Geometry check sheet. Reference: the model listing, model coordinates, mm. Coordinates: 2 decimals unless noted, no trailing zeros. Write each loop counter-clockwise with the first axis right and the second up, starting at its lowest first coordinate (ties: lowest second). Pieces come first, ordered by that corner, then holes. Notation, with made-up numbers: (16, -29.75) -> (27, -29.75) arc R19 ccw to (27, 3.25) -> close; hole circle Ø8 at (53, 66.25). An arc over 180 degrees is marked (long way). One line per question, with ' | ' between items.
from build123d import *

# Parameters (mm, degrees)
F0_W     = 152.4
F0_H     = 114.3
F0_R     = 9.525
F1_DEPTH = 6.35
F2_R     = 12.7


with BuildPart() as f1:
    # F0 (on Top) → F1 (new body)
    with BuildSketch(Plane.XY):
        Rectangle(F0_W, F0_H)
        with BuildLine():
            Line((-8.885304, -47.623662), (-9.393304, -47.623662))
            Line((-9.393304, -47.623662), (-59.177304, -47.623662))
            ThreePointArc((-59.177304, -47.623662), (-59.307662, -47.626338), (-59.43802, -47.623662))
            Line((-59.43802, -47.623662), (-59.685304, -47.623662))
            ThreePointArc((-59.685304, -47.623662), (-59.815662, -47.626338), (-59.94602, -47.623662))
            Line((-59.94602, -47.623662), (-60.193304, -47.623662))
            ThreePointArc((-60.193304, -47.623662), (-63.499331, -44.515193), (-60.323662, -41.273662))
            Line((-60.323662, -41.273662), (-59.815662, -41.273662))
            Line((-59.815662, -41.273662), (-59.307662, -41.273662))
            Line((-59.307662, -41.273662), (-9.393304, -41.273662))
            Line((-9.393304, -41.273662), (-8.885304, -41.273662))
            Line((-8.885304, -41.273662), (-8.377304, -41.273662))
            ThreePointArc((-8.377304, -41.273662), (-5.202304, -44.448662), (-8.377304, -47.623662))
            Line((-8.377304, -47.623662), (-8.885304, -47.623662))
        make_face(mode=Mode.SUBTRACT)
        with BuildLine():
            Line((-8.885304, -34.923662), (-9.393304, -34.923662))
            Line((-9.393304, -34.923662), (-59.177304, -34.923662))
            ThreePointArc((-59.177304, -34.923662), (-59.307662, -34.926338), (-59.43802, -34.923662))
            Line((-59.43802, -34.923662), (-59.685304, -34.923662))
            ThreePointArc((-59.685304, -34.923662), (-59.815662, -34.926338), (-59.94602, -34.923662))
            Line((-59.94602, -34.923662), (-60.193304, -34.923662))
            ThreePointArc((-60.193304, -34.923662), (-63.499331, -31.815193), (-60.323662, -28.573662))
            Line((-60.323662, -28.573662), (-59.815662, -28.573662))
            Line((-59.815662, -28.573662), (-59.307662, -28.573662))
            Line((-59.307662, -28.573662), (-9.393304, -28.573662))
            Line((-9.393304, -28.573662), (-8.885304, -28.573662))
            Line((-8.885304, -28.573662), (-8.377304, -28.573662))
            ThreePointArc((-8.377304, -28.573662), (-5.202304, -31.748662), (-8.377304, -34.923662))
            Line((-8.377304, -34.923662), (-8.885304, -34.923662))
        make_face(mode=Mode.SUBTRACT)
        with BuildLine():
            Line((-8.885304, -22.223662), (-9.393304, -22.223662))
            Line((-9.393304, -22.223662), (-59.177304, -22.223662))
            ThreePointArc((-59.177304, -22.223662), (-59.307662, -22.226338), (-59.43802, -22.223662))
            Line((-59.43802, -22.223662), (-59.685304, -22.223662))
            ThreePointArc((-59.685304, -22.223662), (-59.815662, -22.226338), (-59.94602, -22.223662))
            Line((-59.94602, -22.223662), (-60.193304, -22.223662))
            ThreePointArc((-60.193304, -22.223662), (-63.499331, -19.115193), (-60.323662, -15.873662))
            Line((-60.323662, -15.873662), (-59.815662, -15.873662))
            Line((-59.815662, -15.873662), (-59.307662, -15.873662))
            Line((-59.307662, -15.873662), (-9.393304, -15.873662))
            Line((-9.393304, -15.873662), (-8.885304, -15.873662))
            Line((-8.885304, -15.873662), (-8.377304, -15.873662))
            ThreePointArc((-8.377304, -15.873662), (-5.202304, -19.048662), (-8.377304, -22.223662))
            Line((-8.377304, -22.223662), (-8.885304, -22.223662))
        make_face(mode=Mode.SUBTRACT)
        with BuildLine():
            Line((-8.885304, -9.523662), (-9.393304, -9.523662))
            Line((-9.393304, -9.523662), (-59.177304, -9.523662))
            ThreePointArc((-59.177304, -9.523662), (-59.307662, -9.526338), (-59.43802, -9.523662))
            Line((-59.43802, -9.523662), (-59.685304, -9.523662))
            ThreePointArc((-59.685304, -9.523662), (-59.815662, -9.526338), (-59.94602, -9.523662))
            Line((-59.94602, -9.523662), (-60.193304, -9.523662))
            ThreePointArc((-60.193304, -9.523662), (-63.499331, -6.415193), (-60.323662, -3.173662))
            Line((-60.323662, -3.173662), (-59.815662, -3.173662))
            Line((-59.815662, -3.173662), (-59.307662, -3.173662))
            Line((-59.307662, -3.173662), (-9.393304, -3.173662))
            Line((-9.393304, -3.173662), (-8.885304, -3.173662))
            Line((-8.885304, -3.173662), (-8.377304, -3.173662))
            ThreePointArc((-8.377304, -3.173662), (-5.202304, -6.348662), (-8.377304, -9.523662))
            Line((-8.377304, -9.523662), (-8.885304, -9.523662))
        make_face(mode=Mode.SUBTRACT)
        with Locations((38.1, -31.75)):
            Circle(F0_R, mode=Mode.SUBTRACT)
        with BuildLine():
            Line((-8.885304, 3.176338), (-9.393304, 3.176338))
            Line((-9.393304, 3.176338), (-59.177304, 3.176338))
            ThreePointArc((-59.177304, 3.176338), (-59.307662, 3.173662), (-59.43802, 3.176338))
            Line((-59.43802, 3.176338), (-59.685304, 3.176338))
            ThreePointArc((-59.685304, 3.176338), (-59.815662, 3.173662), (-59.94602, 3.176338))
            Line((-59.94602, 3.176338), (-60.193304, 3.176338))
            ThreePointArc((-60.193304, 3.176338), (-63.499331, 6.284807), (-60.323662, 9.526338))
            Line((-60.323662, 9.526338), (-59.815662, 9.526338))
            Line((-59.815662, 9.526338), (-59.307662, 9.526338))
            Line((-59.307662, 9.526338), (-9.393304, 9.526338))
            Line((-9.393304, 9.526338), (-8.885304, 9.526338))
            Line((-8.885304, 9.526338), (-8.377304, 9.526338))
            ThreePointArc((-8.377304, 9.526338), (-5.202304, 6.351338), (-8.377304, 3.176338))
            Line((-8.377304, 3.176338), (-8.885304, 3.176338))
        make_face(mode=Mode.SUBTRACT)
        with BuildLine():
            Line((-8.885304, 15.876338), (-9.393304, 15.876338))
            Line((-9.393304, 15.876338), (-59.177304, 15.876338))
            ThreePointArc((-59.177304, 15.876338), (-59.307662, 15.873662), (-59.43802, 15.876338))
            Line((-59.43802, 15.876338), (-59.685304, 15.876338))
            ThreePointArc((-59.685304, 15.876338), (-59.815662, 15.873662), (-59.94602, 15.876338))
            Line((-59.94602, 15.876338), (-60.193304, 15.876338))
            ThreePointArc((-60.193304, 15.876338), (-63.499331, 18.984807), (-60.323662, 22.226338))
            Line((-60.323662, 22.226338), (-59.815662, 22.226338))
            Line((-59.815662, 22.226338), (-59.307662, 22.226338))
            Line((-59.307662, 22.226338), (-9.393304, 22.226338))
            Line((-9.393304, 22.226338), (-8.885304, 22.226338))
            Line((-8.885304, 22.226338), (-8.377304, 22.226338))
            ThreePointArc((-8.377304, 22.226338), (-5.202304, 19.051338), (-8.377304, 15.876338))
            Line((-8.377304, 15.876338), (-8.885304, 15.876338))
        make_face(mode=Mode.SUBTRACT)
        with BuildLine():
            Line((-8.885304, 28.576338), (-9.393304, 28.576338))
            Line((-9.393304, 28.576338), (-59.177304, 28.576338))
            ThreePointArc((-59.177304, 28.576338), (-59.307662, 28.573662), (-59.43802, 28.576338))
            Line((-59.43802, 28.576338), (-59.685304, 28.576338))
            ThreePointArc((-59.685304, 28.576338), (-59.815662, 28.573662), (-59.94602, 28.576338))
            Line((-59.94602, 28.576338), (-60.193304, 28.576338))
            ThreePointArc((-60.193304, 28.576338), (-63.499331, 31.684807), (-60.323662, 34.926338))
            Line((-60.323662, 34.926338), (-59.815662, 34.926338))
            Line((-59.815662, 34.926338), (-59.307662, 34.926338))
            Line((-59.307662, 34.926338), (-9.393304, 34.926338))
            Line((-9.393304, 34.926338), (-8.885304, 34.926338))
            Line((-8.885304, 34.926338), (-8.377304, 34.926338))
            ThreePointArc((-8.377304, 34.926338), (-5.202304, 31.751338), (-8.377304, 28.576338))
            Line((-8.377304, 28.576338), (-8.885304, 28.576338))
        make_face(mode=Mode.SUBTRACT)
        with BuildLine():
            Line((-8.885304, 41.276338), (-9.393304, 41.276338))
            Line((-9.393304, 41.276338), (-59.177304, 41.276338))
            ThreePointArc((-59.177304, 41.276338), (-59.307662, 41.273662), (-59.43802, 41.276338))
            Line((-59.43802, 41.276338), (-59.685304, 41.276338))
            ThreePointArc((-59.685304, 41.276338), (-59.815662, 41.273662), (-59.94602, 41.276338))
            Line((-59.94602, 41.276338), (-60.193304, 41.276338))
            ThreePointArc((-60.193304, 41.276338), (-63.499331, 44.384807), (-60.323662, 47.626338))
            Line((-60.323662, 47.626338), (-59.815662, 47.626338))
            Line((-59.815662, 47.626338), (-59.307662, 47.626338))
            Line((-59.307662, 47.626338), (-9.393304, 47.626338))
            Line((-9.393304, 47.626338), (-8.885304, 47.626338))
            Line((-8.885304, 47.626338), (-8.377304, 47.626338))
            ThreePointArc((-8.377304, 47.626338), (-5.202304, 44.451338), (-8.377304, 41.276338))
            Line((-8.377304, 41.276338), (-8.885304, 41.276338))
        make_face(mode=Mode.SUBTRACT)
        with Locations((38.1, 0)):
            Circle(F0_R, mode=Mode.SUBTRACT)
        with Locations((38.1, 31.75)):
            Circle(F0_R, mode=Mode.SUBTRACT)
    extrude(amount=F1_DEPTH)

    # F2
    f2_edges = [f1.edges().sort_by_distance(p)[0] for p in [
        (-76.2, 57.15, 3.175),
        (-76.2, -57.15, 3.175),
        (76.2, 57.15, 3.175),
        (76.2, -57.15, 3.175),
    ]]
    fillet(f2_edges, radius=F2_R)


solid = f1.part
1. Material ranges on line 1 (Y direction, x = 38.1, z = 5.25) (3 decimals); line 2 (X direction, y = 3, z = 1.25); line 3 (X direction, y = 30, z = 4.5), recorded low to high. Write a range as from..to.
Worked answers:
line 1: -57.15..-41.275, -22.225..-9.525, 9.525..22.225, 41.275..57.15 | line 2: -76.2..29.06, 47.14..76.2 | line 3: -76.2..-62.97, -5.73..28.74, 47.46..76.2
2. Cross-section at B-B on y = 19.05. Record the boundary of the cut face in (x, z), and give its area (3 significant figures).
Worked answers:
outline: (-76.2, 0) -> (-63.5, 0) -> (-63.5, 6.35) -> (-76.2, 6.35) -> close; (-5.2, 0) -> (76.2, 0) -> (76.2, 6.35) -> (-5.2, 6.35) -> close | area: 598 mm²
3. Cross-section at A-A on y = 31.75. Record the boundary of the cut face in (x, z) (3 decimals).
Worked answers:
outline: (-76.2, 0) -> (-63.5, 0) -> (-63.5, 6.35) -> (-76.2, 6.35) -> close; (-5.202, 0) -> (28.575, 0) -> (28.575, 6.35) -> (-5.202, 6.35) -> close; (47.625, 0) -> (76.2, 0) -> (76.2, 6.35) -> (47.625, 6.35) -> close
4. Go/stop test with a flat-tipped pin: P1, Ø15, axis at x = 38.1, y = -31.75, coming from the +Z side. Record where the tip stops, or that it passes through.
Worked answers:
P1: through
5. Cross-section at D-D on z = 3.5. Give the number of separate pieces and of enclosed holes in the cut face, and give its area (3 significant figures).
Worked answers:
separate pieces: 1 | enclosed holes: 11 | area: 13,500 mm²
6. Cross-section at C-C on x = 40. Record the boundary of the cut face in (y, z).
Worked answers:
outline: (-57.15, 0) -> (-41.08, 0) -> (-41.08, 6.35) -> (-57.15, 6.35) -> close; (-22.42, 0) -> (-9.33, 0) -> (-9.33, 6.35) -> (-22.42, 6.35) -> close; (9.33, 0) -> (22.42, 0) -> (22.42, 6.35) -> (9.33, 6.35) -> close; (41.08, 0) -> (57.15, 0) -> (57.15, 6.35) -> (41.08, 6.35) -> close
7. Mould release check, pull along Y, two halves, no side actions. Record for faces 1 (the face through (-33, -22.224, 3)), 2 (the face through (72.38, 53.53, 3.22)), 3 (the face through (72.38, -53.53, 3.22)): released by +Y, released by -Y, zero draft, split by the parting line, or undercut.
Worked answers:
face 1: undercut | face 2: released by +Y | face 3: released by -Y
